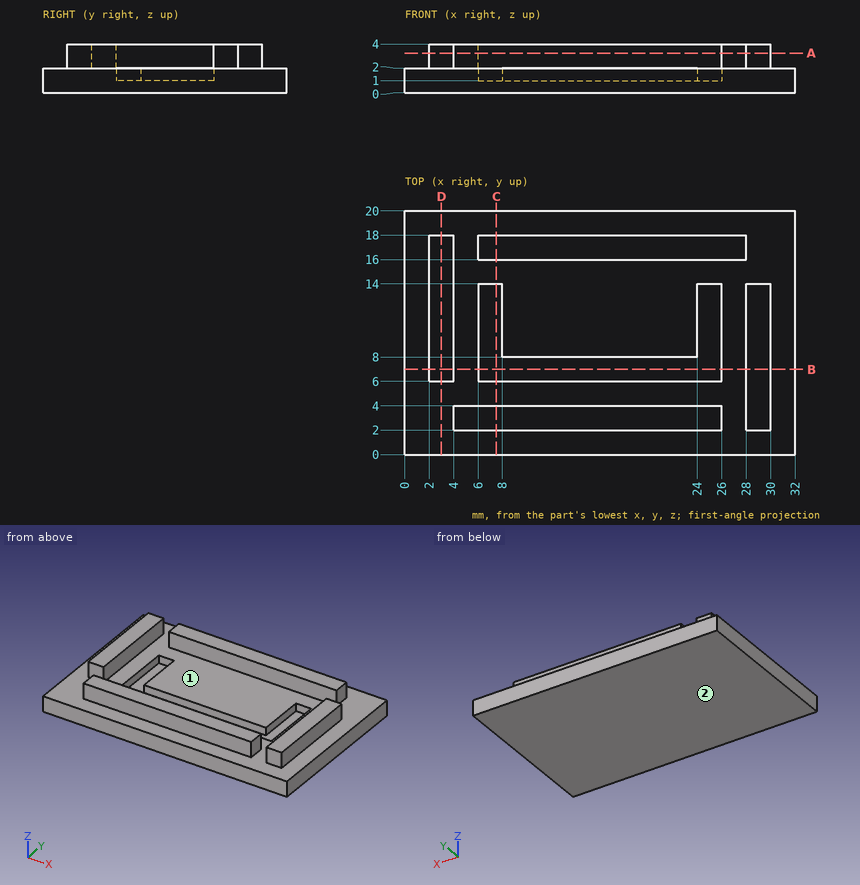
Verification items for this drawing (mm, ordinates from the low corner). Coordinates: 2 decimals unless noted, no trailing zeros. Loops run counter-clockwise (first coordinate to the right, second up) from the corner with the lowest first, then second, coordinate; pieces in that order, holes last. Notation, with made-up numbers: (-38.75, 79) - (9.25, 79) arc R24 cw to (9.25, 95) - close; hole circle Ø9 at (59, 35). An arc over 180 degrees is marked (long way). One line per item, written item: value. Start each with the question number.
(1) Cross-section at A-A on z = 3.25. Enter the section's corners in (x, y), plus the area to 3 significant figures.
(2) Mould release check, pull along Y, two halves, no side actions. Record for the marked faces 1 and 2: released by +Y, released by -Y, zero draft, split by the parting line, or undercut.
(3) Depth check by flat-ended pin: P1, Ø4, axis at x = 15.5, y = 10, coming from the +Z side; P2, Ø1, axis at x = 19, y = 10, coming from the -Z side; P3, Ø0.6, axis at x = 13, z = 2.5, coming from the -Y side; P4, Ø2, axis at x = 18, z = 3.5, coming from the +Y side. Enter the tip coordinate at first touch or a pass-through.
(4) Material ranges on line 1 (X direction, y = 8.5, z = 1.3); line 2 (Y direction, x = 13.5, z = 1.6); line 3 (X direction, y = 13.75, z = 2.2), recorded low to high. Write a range as [from, to].
(5) Cross-section at C-C on x = 7.5. Enter the section's corners in (y, z).
(6) Cross-section at D-D on x = 3. Enter the section's corners in (y, z).
(7) Cross-section at B-B on y = 7. Enter the section's corners in (x, z).
Results below:
1. outline: (2, 6) - (4, 6) - (4, 18) - (2, 18) - close; (4, 2) - (26, 2) - (26, 4) - (4, 4) - close; (6, 16) - (28, 16) - (28, 18) - (6, 18) - close; (28, 2) - (30, 2) - (30, 14) - (28, 14) - close
1. area: 136 mm2
2. face 1: undercut
2. face 2: zero draft
3. P1: stops at z = 2
3. P2: stops at z = 0
3. P3: stops at y = 2
3. P4: stops at y = 18
4. line 1: x = [0, 6], [8, 24], [26, 32]
4. line 2: y = [0, 6], [8, 20]
4. line 3: x = [2, 4], [28, 30]
5. outline: (0, 0) - (20, 0) - (20, 2) - (18, 2) - (18, 4) - (16, 4) - (16, 2) - (14, 2) - (14, 1) - (6, 1) - (6, 2) - (4, 2) - (4, 4) - (2, 4) - (2, 2) - (0, 2) - close
6. outline: (0, 0) - (20, 0) - (20, 2) - (18, 2) - (18, 4) - (6, 4) - (6, 2) - (0, 2) - close
7. outline: (0, 0) - (32, 0) - (32, 2) - (30, 2) - (30, 4) - (28, 4) - (28, 2) - (26, 2) - (26, 1) - (6, 1) - (6, 2) - (4, 2) - (4, 4) - (2, 4) - (2, 2) - (0, 2) - close
